Could you check a few things on this model? Use its own coordinates, in mm. Give positions to 0.01 mm unless a question says otherwise; leave off trailing zeros. Order: outer loops, then holes, each group sorted by start corner. A loop starts at its lowest first (then second) coordinate and runs counter-clockwise, first axis right, second up.
from build123d import *

# Parameters (mm, degrees)
SKETCH1_W           = 120
SKETCH1_H           = 120
SKETCH1_R           = 2.55
SKETCH1_R_2         = 20
BOSS_EXTRUDE1_DEPTH = 5
SKETCH2_W           = 120
SKETCH2_H           = 5
BOSS_EXTRUDE2_DEPTH = 280


with BuildPart() as part:
    # Sketch1 → Boss-Extrude1 (new body)
    with BuildSketch(Plane(origin=(0, 0, 0), x_dir=(1, 0, 0), z_dir=(0, 1, 0))):
        Rectangle(SKETCH1_W, SKETCH1_H)
        with Locations(Location((-25.000001015, -25.000001015, 0), (0, 0, 270))):
            Circle(SKETCH1_R, mode=Mode.SUBTRACT)
        with Locations(Location((24.999998985, -24.999998985, 0), (0, 0, 270))):
            Circle(SKETCH1_R, mode=Mode.SUBTRACT)
        with Locations(Location((25.000001015, 25.000001015, 0), (0, 0, 270))):
            Circle(SKETCH1_R, mode=Mode.SUBTRACT)
        with Locations(Location((-24.999998985, 24.999998985, 0), (0, 0, 270))):
            Circle(SKETCH1_R, mode=Mode.SUBTRACT)
        with Locations(Location((0, 0, 0), (0, 0, 270))):
            Circle(SKETCH1_R_2, mode=Mode.SUBTRACT)
    extrude(amount=BOSS_EXTRUDE1_DEPTH)

    # Sketch2 → Boss-Extrude2 (add)
    with BuildSketch(Plane.XY.offset(60)):
        with Locations((0, 2.5)):
            Rectangle(SKETCH2_W, SKETCH2_H)
    extrude(amount=BOSS_EXTRUDE2_DEPTH)


solid = part.part
Item 1: Imagine slicing it at A-A on z = 0. List the corners of the cut face in (x, y) for me, then the cut area to 3 significant figures.
Findings:
outline: (-60, 0) - (-20, 0) - (-20, 5) - (-60, 5) - close; (20, 0) - (60, 0) - (60, 5) - (20, 5) - close
area: 400 mm2
Item 2: Please list where these lines run through material, in increasing order: line 1 along X through (y, z) = (4.85, 24.5); line 2 along Z through (x, y) = (10, 3.2); line 3 along Z through (x, y) = (13, 4).
Findings:
line 1: x = -60 to -27.5, -22.5 to 22.5, 27.5 to 60
line 2: z = -60 to -17.32, 17.32 to 340
line 3: z = -60 to -15.2, 15.2 to 340
Item 3: We'd pull the mould along X, two halves only. Please class faces 1 (the cylindrical face through (-19.524, 2.465, -4.336)), 2 (the flat face through (-1, 0, 137)): +X half, -X half, draft (parallel to the pull), parting line (faces both ways), or undercut.
Findings:
face 1: undercut
face 2: draft
Item 4: Imagine slicing it at C-C on x = -14. List the corners of the cut face in (y, z) for me, then the cut area to 3 significant figures.
Findings:
outline: (0, -60) - (5, -60) - (5, -14.28) - (0, -14.28) - close; (0, 14.28) - (5, 14.28) - (5, 340) - (0, 340) - close
area: 1,860 mm2
Item 5: Imagine slicing it at B-B on y = 0.85. List the corners of the cut face in (x, z) for me.
Findings:
outline: (-60, -60) - (60, -60) - (60, 340) - (-60, 340) - close; hole circle Ø5.1 at (-25, -25); hole circle Ø5.1 at (-25, 25); hole circle Ø40 at (0, 0); hole circle Ø5.1 at (25, -25); hole circle Ø5.1 at (25, 25)
Item 6: For pin 1 (24 mm diameter, centred on x = 0, z = 0, fed in from -Y), with a flat end and sliding along its axis, tell me the tip position at first contact or that it passes through.
Findings:
pin 1: passes through
